The listing builds one solid part. Answer for the finished solid, in the listing's coordinates (mm). Give positions to 0.01 mm unless a question says otherwise; leave off trailing zeros. Write each loop counter-clockwise with the first axis right and the second up, starting at its lowest first coordinate (ties: lowest second). Pieces come first, ordered by that corner, then holes. Notation, with made-up numbers: (25, 57.25) - (32, 57.25) arc R11 ccw to (32, 78.25) - close; hole circle Ø3 at (77, 56.25). An arc over 180 degrees is marked (long way). Answer as CSV lines item,"result". Start each with the question number.
(1) Find section B-B (z = 5.2). State how many separate pieces and enclosed holes the cut face has, then the cut area to 3 significant figures.
(2) For a pull along X with two mould halves and no side action, classify faces 1 (the face through (9.738, -65.208, 2.958)), 2 (the face through (-17.766, -14.356, 2.812)), 3 (the face through (-15, -14, 6)) as pulls with the +X half, pulls with the -X half, needs draft (parallel to the pull), parting line crosses it, or undercut.
(3) Straight lines are drawn through the part: probe 1 along X at (y, z) = (-12.5, 3.5); probe 2 along Y at (x, z) = (-20, 2.2); probe 3 along X at (y, z) = (-50, 1.4). For each, find the intervals that lie inside material, in ascending order.
(4) Find section A-A (y = 0). Write down the section's boundary in (x, z).
Autodesk Inventor part; units mm, degrees
ref_plane "YZ Plane" through (0, 0, 0) normal (1, 0, 0) x (0, 1, 0)
ref_plane "XZ Plane" through (0, 0, 0) normal (0, 1, 0) x (-1, 0, 0)
ref_plane "XY Plane" through (0, 0, 0) normal (0, 0, 1) x (1, 0, 0)
ref_plane "Work Plane1" through (0, 0, 0) normal (0, 0, 1) x (1, 0, 0)
sketch "Sketch1" plane through (0, 0, 0) normal (0, 0, 1) x (1, 0, 0)
  line L0 (10.8382, -62.5107) -> (10.8382, 0.6668)
  line L1 (6.9805, -66.3684) -> (-18, -66.3684)
  line L2 (10.8382, -5.7047) -> (9.6808, -5.7047) construction
  line L3 (10.8382, 0.6668) -> (10.8382, 2.1422)
  line L4 (-40.1739, 0.853) -> (-40.1739, 2.1422)
  line L5 (6.9805, 6) -> (-36.3161, 6)
  circle A0 centre (-3.9646, 0) radius 1.45
  circle A1 centre (-32.0354, 0) radius 1.45
  circle A2 centre (-18, -62.5107) radius 2.45
  arc A3 (-20.665, -65.3) -> (-18, -66.3684) centre (-18, -62.5107) ccw
  arc A4 (6.9805, -66.3684) -> (10.8382, -62.5107) centre (6.9805, -62.5107) ccw
  arc A5 (-36.3161, 6) -> (-40.1739, 2.1422) centre (-36.3161, 2.1422) ccw
  arc A6 (10.8382, 2.1422) -> (6.9805, 6) centre (6.9805, 2.1422) ccw
  line L6 (-18, -66.3684) -> (-35.1739, -66.3684)
  line L7 (-40.1739, -61.3684) -> (-40.1739, 0.853)
  arc A7 (-40.1739, -61.3684) -> (-35.1739, -66.3684) centre (-35.1739, -61.3684) ccw
  point P0 (0, 0)
  point P1 (10.8382, 6)
  point P2 (-40.1739, 6)
  dimension "d6" = 2.9
  dimension "d7" = 2.9
  dimension "d32" = 90
  dimension "d46" = 5
  dimension "d47" = 62.5107
  dimension "d48" = 28.0709
  dimension "d49" = 64.067
extrude "Extrusion1" add sketch "Sketch1" along normal blind 6
sketch "Sketch8" plane through (0, 0, 6) normal (0, 0, 1) x (1, 0, 0)
  circle A0 centre (-18, -62.5107) radius 2.45
  circle A1 centre (-32.0354, 0) radius 1.45
  circle A2 centre (-3.9646, 0) radius 1.45
  line L0 (-35.1739, -66.3684) -> (6.9805, -66.3684)
  arc A3 (6.9805, -66.3684) -> (10.8382, -62.5107) centre (6.9805, -62.5107) ccw
  line L1 (10.8382, -62.5107) -> (10.8382, 2.1422)
  arc A4 (10.8382, 2.1422) -> (6.9805, 6) centre (6.9805, 2.1422) ccw
  line L2 (6.9805, 6) -> (-36.3161, 6)
  arc A5 (-36.3161, 6) -> (-40.1739, 2.1422) centre (-36.3161, 2.1422) ccw
  line L3 (-40.1739, 2.1422) -> (-40.1739, -61.3684)
  arc A6 (-40.1739, -61.3684) -> (-35.1739, -66.3684) centre (-35.1739, -61.3684) ccw
  circle A7 centre (-14.0967, -30.8778) radius 16.7364
  line L4 (4.4033, -49.3778) -> (-32.5967, -49.3778)
  line L5 (-32.5967, -49.3778) -> (-32.5967, -12.3778)
  line L6 (-32.5967, -12.3778) -> (4.4033, -12.3778)
  line L7 (4.4033, -12.3778) -> (4.4033, -49.3778)
  line L8 (4.4033, -49.3778) -> (-32.5967, -12.3778) construction
  line L9 (-32.5967, -49.3778) -> (4.4033, -12.3778) construction
  circle A8 centre (-32.5967, -12.3778) radius 2.45
  circle A9 centre (4.4033, -12.3778) radius 2.45
  circle A10 centre (4.4033, -49.3778) radius 2.45
  circle A11 centre (-32.5967, -49.3778) radius 2.45
  point P0 (0, 0)
  dimension "d52" = 37
  dimension "d53" = 37
  dimension "d54" = 4.9
  dimension "d55" = 4.9
  dimension "d56" = 4.9
  dimension "d57" = 4.9
extrude "Extrusion7" cut sketch "Sketch8" against normal through all contours A7 | A11 L5 L4 | L4 L5 A11 | A10 L7 L4 | L4 L7 A10 | A8 L6 L5 | L5 L6 A8 | A9 L6 L7 | L7 L6 A9
chamfer "Chamfer3" distance 3 angle 45 1 edges at (-30.8332, -30.8778, 0)
properties part number "cellSTORM_inverted_chiptray_v0"
Result set:
1,separate pieces,"1"
1,enclosed holes,"8"
1,area,"2,690 mm^2"
2,face 1,"pulls with the +X half"
2,face 2,"undercut"
2,face 3,"needs draft"
3,probe 1,"-40.17 to -35.04, -30.15 to 1.96, 6.85 to 10.84"
3,probe 2,"-66.37 to -63.93, -61.1 to -47.39, -14.36 to 6"
3,probe 3,"-40.17 to -34.97, -30.23 to 2.03, 6.77 to 10.84"
4,outline,"(-40.17, 0) - (-33.49, 0) - (-33.49, 6) - (-40.17, 6) - close; (-30.59, 0) - (-5.41, 0) - (-5.41, 6) - (-30.59, 6) - close; (-2.51, 0) - (10.84, 0) - (10.84, 6) - (-2.51, 6) - close"
